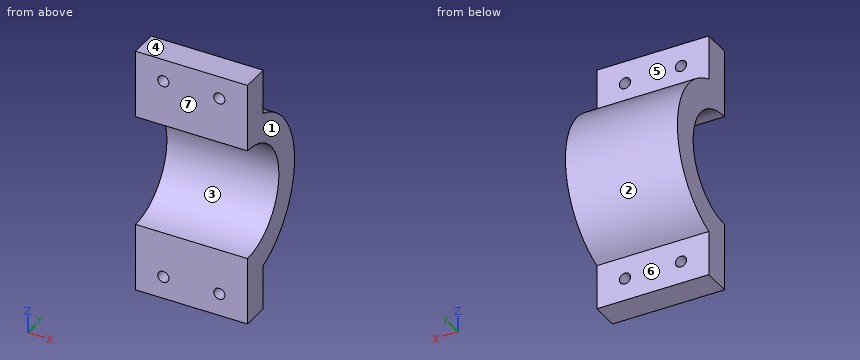
Autodesk Inventor part; units mm, degrees
ref_plane "YZ Plane" through (0, 0, 0) normal (1, 0, 0) x (0, 1, 0)
ref_plane "XZ Plane" through (0, 0, 0) normal (0, 1, 0) x (-1, 0, 0)
ref_plane "XY Plane" through (0, 0, 0) normal (0, 0, 1) x (1, 0, 0)
sketch "Sketch1" plane through (0, 0, 0) normal (1, 0, 0) x (0, 1, 0)
  arc A0 (0, -20) -> (0, 20) centre (0, 0) ccw
  arc A1 (10, -28.2843) -> (10, 28.2843) centre (0, 0) ccw
  line L0 (10, 44.2843) -> (0, 44.2843)
  line L1 (0, -44.2843) -> (10, -44.2843)
  line L2 (10, -44.2843) -> (10, -28.2843)
  line L3 (10, 28.2843) -> (10, 44.2843)
  line L4 (0, 44.2843) -> (0, 20)
  line L5 (0, -20) -> (0, -44.2843)
  line L6 (0, 44.2843) -> (0, 20)
  line L7 (0, -20) -> (0, -44.2843)
  dimension "d2" = 30
  dimension "d3" = 20
  dimension "d5" = 10
  dimension "d6" = 10
  dimension "d11" = 16
  dimension "d12" = 16
extrude "Extrusion1" add sketch "Sketch1" along normal blind 40
sketch "Sketch4" plane through (0, 10, 44.2843) normal (0, 1, 0) x (1, 0, 0)
  line L0 (0, 0) -> (0, 24.2843) construction
  line L1 (0, 8) -> (0, -32) construction
  line L2 (0, 8) -> (40.1355, 8) construction
  line L3 (0, 0) -> (40, 0)
  line L4 (10, 0) -> (-6, 0)
  line L5 (10, 0) -> (10, 16.0426) construction
  line L6 (30, 0) -> (30, 16) construction
  line L7 (0, 16) -> (40, 16)
  point P0 (0, 44.2843)
  dimension "d13" = 40
  dimension "d14" = 16
sketch "Sketch5" plane through (0, 10, 44.2843) normal (0, 1, 0) x (1, 0, 0)
  point P0 (0, 44.2843)
  point P1 (9.9387, 7.9868)
  point P2 (29.9524, 8.0308)
hole "Hole1" at (9.9387, 10, 36.2975) at (29.9524, 10, 36.2535) direction (0, -1, 0) diameter 4 end through all
thread "Thread1"
thread "Thread2"
mirror "Mirror1" about plane through (0, 0, 0) normal (0, 0, 1) of "Hole1"
thread "Thread3"
thread "Thread4"
properties part number "U_bracket"
The model under review builds one solid part; all positions refer to its coordinate system, in mm. Face numbers are marked on the shaded views. A direction names the side the tool comes from. Give positions to 0.01 mm unless a question says otherwise; leave off trailing zeros. Loops run counter-clockwise (first coordinate to the right, second up) from the corner with the lowest first, then second, coordinate; pieces in that order, holes last. Notation, with made-up numbers: (-9.75, 22.25) -> (6.25, 22.25) arc R23 ccw to (6.25, 51.25) -> close; hole circle Ø1 at (16, 43.25). An arc over 180 degrees is marked (long way). Answer as a JSON object with one key per item and string values. Group by question number.
Q1. Take a section at D-D (x = 29). Write out the cut boundary in (y, z).
Q2. Insertion check: pin 1 (1 mm diameter, centred on x = 11.5, z = -24, fed in from +Y); pin 2 (5 mm diameter, centred on x = 9.94, z = 36.3, fed in from +Y); pin 3 (6 mm diameter, centred on x = 17.5, z = 14.5, fed in from +Y); pin 4 (3.5 mm diameter, centred on x = 9.94, z = -36.3, fed in from +Y). Each pin has a flat end and moves straight along its axis. Give the tip position at first contact, or say it passes through.
Q3. Take a section at B-B (x = 13.5). Write out the cut boundary in (y, z), plus the area to 3 significant figures.
Q4. Take a section at A-A (y = 19). Write out the cut boundary in (x, z) (3 decimals), plus the area to 3 significant figures.
Q5. Wall thickness on line 1 along X through (y, z) = (7.5, 35); line 2 along Z through (x, y) = (30, 7.5); line 3 along X through (y, z) = (6, 38): over which ranges is each line inside the solid? List them lowest first.
Q6. Take a section at C-C (z = 0). Write out the cut boundary in (x, y).
Q7. Draft analysis for pull direction Z (two halves, no side actions). For the marked faces 1, 2, 3 and 4, state which applies: pulls with the +Z half, pulls with the -Z half, needs draft (parallel to the pull), parting line crosses it, or undercut.
Q8. Tool access review of the marked faces 5, 6 and 7: name each direction out of +Z, -Z, +X, -X, +Y, -Y from which nothing blocks a thin tool from reaching the whole face with its end or side.
Answer below:
{
 "1": {"outline": "(0, -44.28) -> (10, -44.28) -> (10, -38.01) -> (0, -38.01) -> close; (0, -34.49) -> (10, -34.49) -> (10, -28.28) arc R30 ccw to (10, 28.28) -> (10, 34.49) -> (0, 34.49) -> (0, 20) arc R20 cw to (0, -20) -> close; (0, 38.01) -> (10, 38.01) -> (10, 44.28) -> (0, 44.28) -> close"},
 "2": {"pin 1": "stops at y = 18.65", "pin 2": "stops at y = 10", "pin 3": "stops at y = 27.71", "pin 4": "passes through"},
 "3": {"outline": "(0, -44.28) -> (10, -44.28) -> (10, -28.28) arc R30 ccw to (10, 28.28) -> (10, 44.28) -> (0, 44.28) -> (0, 20) arc R20 cw to (0, -20) -> close", "area": "1,080 mm2"},
 "4": {"outline": "(0, -23.216) -> (40, -23.216) -> (40, -6.245) -> (0, -6.245) -> close; (0, 6.245) -> (40, 6.245) -> (40, 23.216) -> (0, 23.216) -> close", "area": "1,360 mm2"},
 "5": {"line 1": "x = 0 to 8.42, 11.46 to 28.39, 31.51 to 40", "line 2": "z = -44.28 to -38.25, -34.25 to -18.54, 18.54 to 34.25, 38.25 to 44.28", "line 3": "x = 0 to 8.89, 10.99 to 28.98, 30.93 to 40"},
 "6": {"outline": "(0, 20) -> (40, 20) -> (40, 30) -> (0, 30) -> close"},
 "7": {"face 1": "needs draft", "face 2": "parting line crosses it", "face 3": "undercut", "face 4": "pulls with the +Z half"},
 "8": {"face 5": "+Z, +X, -X, +Y", "face 6": "-Z, +X, -X, +Y", "face 7": "+Z, -Z, +X, -X, -Y"}
}
